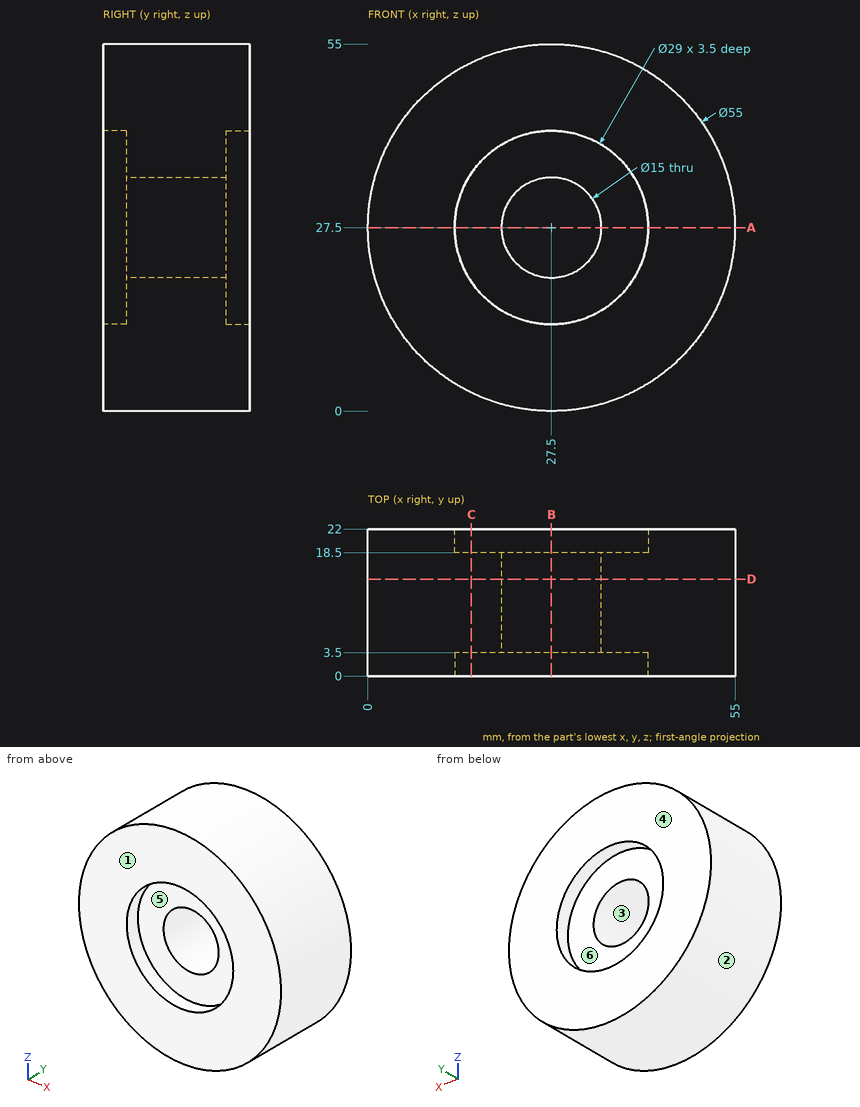
Drawing for the job (mm, zero at the part's lowest x, y, z). A direction names the side the tool comes from. Coordinates: 2 decimals unless noted, no trailing zeros. Order: outer loops, then holes, each group sorted by start corner. A loop starts at its lowest first (then second) coordinate and runs counter-clockwise, first axis right, second up. Notation, with made-up numbers: (20, -34.5) -> (28, -34.5) arc R30 cw to (28, -7.5) -> close; hole circle Ø5 at (44.5, 68). An arc over 180 degrees is marked (long way). Return JSON: item names as keys, results as strings.
Item 1: Slice it at C-C (x = 15.5). Write the cut outline in (y, z).
Model answer:
{"outline": "(0, 2.76) -> (22, 2.76) -> (22, 19.36) -> (18.5, 19.36) -> (18.5, 35.64) -> (22, 35.64) -> (22, 52.24) -> (0, 52.24) -> (0, 35.64) -> (3.5, 35.64) -> (3.5, 19.36) -> (0, 19.36) -> close"}
Item 2: 3-axis set-ups, long thin cutter, end or side, ignore diameter. For the marked faces 4, 5 and 6: which of +Z, -Z, +X, -X, +Y, -Y reach the whole face in a straight line?
Model answer:
{"face 4": "+Z, -Z, +X, -X, +Y", "face 5": "-Y", "face 6": "+Y"}
Item 3: Wall check: line 1 along Z through (x, y) = (27.5, 11.75); line 2 along Z through (x, y) = (27.5, 1.45); line 3 along X through (y, z) = (5.5, 28). Give the ranges that are in metal, low to high. Write a range as from..to.
Model answer:
{"line 1": "z = 0..20, 35..55", "line 2": "z = 0..13, 42..55", "line 3": "x = 0..20.02, 34.98..55"}
Item 4: Slice it at A-A (z = 27.5). Write the cut outline in (x, y), then the cut area to 3 significant figures.
Model answer:
{"outline": "(0, 0) -> (13, 0) -> (13, 3.5) -> (20, 3.5) -> (20, 18.5) -> (13, 18.5) -> (13, 22) -> (0, 22) -> close; (35, 3.5) -> (42, 3.5) -> (42, 0) -> (55, 0) -> (55, 22) -> (42, 22) -> (42, 18.5) -> (35, 18.5) -> close", "area": "782 mm²"}
Item 5: Slice it at B-B (x = 27.5). Write the cut outline in (y, z).
Model answer:
{"outline": "(0, 0) -> (22, 0) -> (22, 13) -> (18.5, 13) -> (18.5, 20) -> (3.5, 20) -> (3.5, 13) -> (0, 13) -> close; (0, 42) -> (3.5, 42) -> (3.5, 35) -> (18.5, 35) -> (18.5, 42) -> (22, 42) -> (22, 55) -> (0, 55) -> close"}
Item 6: Mould opens along X. For the marked faces 1, 2 and 3 say: pulls with the +X half, pulls with the -X half, needs draft (parallel to the pull), parting line crosses it, or undercut.
Model answer:
{"face 1": "needs draft", "face 2": "parting line crosses it", "face 3": "undercut"}
Item 7: Pin check, flat tips, straight feed: P1, Ø17.5, axis at x = 27.5, z = 27.5, coming from the +Y side; P2, Ø5, axis at y = 4, z = 32, coming from the -X side; P3, Ø1.5, axis at x = 15.5, y = 6, coming from the -Z side. Stop position of each tip, or through.
Model answer:
{"P1": "stops at y = 18.5", "P2": "stops at x = 0.07", "P3": "stops at z = 2.41"}
Item 8: Slice it at D-D (y = 14.5). Write the cut outline in (x, z).
Model answer:
{"outline": "circle Ø55 at (27.5, 27.5); hole circle Ø15 at (27.5, 27.5)"}
